For this review, take the finished solid that the model builds, in its own axes (mm). A direction names the side the tool comes from. Round coordinates to 2 decimals unless told otherwise and drop trailing zeros. Write each loop counter-clockwise with the first axis right and the second up, starting at its lowest first coordinate (ties: lowest second). Pieces come first, ordered by that corner, then holes. Notation, with made-up numbers: M -17.75,27.25 L 0.25,27.25 A18 ccw 0.25,32.25 Z; hole C 56,70.25 d3. An arc over 180 degrees is marked long. Use one line per item in the form item = value. Start each with the question number.
Item 1: Add section B-B (z = -22). State the section outline as (x, y) points.
Item 2: Add section D-D (x = -6.5). State the section outline as (y, z) points, and give its area (3 significant figures).
Item 3: For faces 4 (the flat face through (-17, -4, -15)), 5 (the cylindrical face through (0.224, 18.859, 1.203)), 6 (the cylindrical face through (0.2, 20.9, -1)), list the 3-axis set-ups (+Z, -Z, +X, -X, +Y, -Y) from which the entire face can be reached by the end or side of a thin tool; tool diameter is ignored.
Item 4: Draft analysis for pull direction Y (two halves, no side actions). For faces 1 (the flat face through (0, -16, -2)), 2 (the cylindrical face through (-1.08, -4.88, 41.52)), 3 (the flat face through (-18, 16, -17)), state which applies: released by +Y, released by -Y, zero draft, split by the parting line, or undercut.
Item 5: Add section A-A (y = 0). Count the separate pieces of the cut face and the enclosed holes in it, and give its area (3 significant figures).
Item 6: Add section C-C (y = 15). State the section outline as (x, z) points, and give its area (3 significant figures).
Item 7: For line 1 (Z direction, x = -11, y = -2); line 2 (Y direction, x = -18, z = -22); line 3 (X direction, y = 5, z = -6.5), list the stretches that pass through material, from the lowest coordinate up. Write a range as [from, to].
Item 8: For P1, Ø2, axis at x = -14, z = 13.5, coming from the -Y side; P2, Ø1, axis at x = -8, z = -1, coming from the +Y side; P3, Ø1.5, axis at x = 7.5, y = 3.5, coming from the -Z side, all flat-tipped, find the tip position at first contact; note any pin that passes through.
from build123d import *

# Parameters (mm, degrees)
SKETCH1_W                      = 32
SKETCH1_H                      = 32
BASE_FLANGE1_DEPTH             = 3
KENAR_FLAN_1_DEPTH             = 32
KENAR_FLAN_2_DEPTH             = 32
KENAR_FLAN_3_DEPTH             = 32
KENAR_FLAN_4_DEPTH             = 32
SKETCH20_R                     = 5
CUT_EXTRUDE1_DEPTH             = 82.884064384
CUT_EXTRUDE2_REACH             = 65.071
SKETCH21_R                     = 7.5
CUT_EXTRUDE2_DIRECTION_2_DEPTH = 64.071388125


# Sheet-metal steps are written as plain solids
with BuildPart() as part:
    # Sketch1 → Base-Flange1 (new body)
    with BuildSketch(Plane.XY):
        Rectangle(SKETCH1_W, SKETCH1_H)
    extrude(amount=-BASE_FLANGE1_DEPTH)

    # Kenar-Flanş1 section (across the edge) → Kenar-Flanş1 (add)
    with BuildSketch(Plane(origin=(16, 20, 0), x_dir=(0, -1, 0), z_dir=(-1, 0, 0))):
        with BuildLine():
            Line((-3, 4), (-3, 36))
            Line((-3, 36), (0, 36))
            Line((0, 36), (0, 4))
            ThreePointArc((0, 4), (1.171572875, 1.171572875), (4, 0))
            Line((4, 0), (4, -3))
            ThreePointArc((4, -3), (-0.949747468, -0.949747468), (-3, 4))
        make_face()
    extrude(amount=KENAR_FLAN_1_DEPTH)

    # Kenar-Flanş2 section (across the edge) → Kenar-Flanş2 (add)
    with BuildSketch(Plane(origin=(16, 20, 40), x_dir=(0, 0, -1), z_dir=(-1, 0, 0))):
        with BuildLine():
            Line((-3, 4), (-3, 36))
            Line((-3, 36), (0, 36))
            Line((0, 36), (0, 4))
            ThreePointArc((0, 4), (1.171572875, 1.171572875), (4, 0))
            Line((4, 0), (4, -3))
            ThreePointArc((4, -3), (-0.949747468, -0.949747468), (-3, 4))
        make_face()
    extrude(amount=KENAR_FLAN_2_DEPTH)

    # Kenar-Flanş3 section (across the edge) → Kenar-Flanş3 (add)
    with BuildSketch(Plane(origin=(-17, -16, -3), x_dir=(1, 0, 0), z_dir=(0, 1, 0))):
        with BuildLine():
            Line((-3, 1), (-3, 30))
            Line((-3, 30), (0, 30))
            Line((0, 30), (0, 1))
            ThreePointArc((0, 1), (0.292893219, 0.292893219), (1, 0))
            Line((1, 0), (1, -3))
            ThreePointArc((1, -3), (-1.828427125, -1.828427125), (-3, 1))
        make_face()
    extrude(amount=KENAR_FLAN_3_DEPTH)

    # Kenar-Flanş4 section (across the edge) → Kenar-Flanş4 (add)
    with BuildSketch(Plane(origin=(17, 16, -3), x_dir=(-1, 0, 0), z_dir=(0, -1, 0))):
        with BuildLine():
            Line((-3, 1), (-3, 30))
            Line((-3, 30), (0, 30))
            Line((0, 30), (0, 1))
            ThreePointArc((0, 1), (0.292893219, 0.292893219), (1, 0))
            Line((1, 0), (1, -3))
            ThreePointArc((1, -3), (-1.828427125, -1.828427125), (-3, 1))
        make_face()
    extrude(amount=KENAR_FLAN_4_DEPTH)

    # Sketch20 → Cut-Extrude1 (cut, through all)
    with BuildSketch(Plane.XY.offset(43)):
        Circle(SKETCH20_R)
    extrude(amount=-CUT_EXTRUDE1_DEPTH, mode=Mode.SUBTRACT)

    # Cut-Extrude2: up to this face of the body (flat: up to its plane)
    cut_extrude2_end = Plane(part.part.faces().sort_by_distance((20, 0, -18.5))[0])
    # Sketch21 → Cut-Extrude2 (cut, up to the picked face)
    with BuildSketch(Plane.ZY.offset(20), mode=Mode.PRIVATE) as cut_extrude2_sk1:
        with Locations((-22, 0)):
            Circle(SKETCH21_R)
    cut_extrude2_tool1 = split(extrude(cut_extrude2_sk1.sketch, amount=-CUT_EXTRUDE2_REACH, mode=Mode.PRIVATE), bisect_by=cut_extrude2_end, keep=Keep.BOTH, mode=Mode.PRIVATE)
    add(cut_extrude2_tool1.solids().sort_by(Axis((-20, 0, -22), (1, 0, 0)))[0], mode=Mode.SUBTRACT)

    # Sketch21 → Cut-Extrude2 direction 2 (cut)
    with BuildSketch(Plane.ZY.offset(20)):
        with Locations((-22, 0)):
            Circle(SKETCH21_R)
    extrude(amount=CUT_EXTRUDE2_DIRECTION_2_DEPTH, mode=Mode.SUBTRACT)


solid = part.part
Calculated:
q1.outline = M -20,-16 L -17,-16 L -17,-7.5 L -20,-7.5 Z; M -20,7.5 L -17,7.5 L -17,16 L -20,16 Z; M 17,-16 L 20,-16 L 20,-7.5 L 17,-7.5 Z; M 17,7.5 L 20,7.5 L 20,16 L 17,16 Z
q2.outline = M -16,-3 L 16,-3 A7 ccw 23,4 L 23,36 A7 ccw 16,43 L -16,43 L -16,40 L 16,40 A4 cw 20,36 L 20,4 A4 cw 16,0 L -16,0 Z
q2.area = 340 mm^2
q3.face_4 = -Z, +Y, -Y
q3.face_5 = +X, -X, -Y
q3.face_6 = -Z, +X, -X, +Y
q4.face_1 = released by -Y
q4.face_2 = undercut
q4.face_3 = released by +Y
q5.separate_pieces = 6
q5.enclosed_holes = 0
q5.area = 240 mm^2
q6.outline = M -20,-33 L -17,-33 L -17,-4 A1 cw -16,-3 L 16,-3 A1 cw 17,-4 L 17,-33 L 20,-33 L 20,-4 A4 ccw 16,0 L -16,0 A4 ccw -20,-4 Z; M -16,40 L 16,40 L 16,43 L -16,43 Z
q6.area = 390 mm^2
q7.line_1 = [-3, 0], [40, 43]
q7.line_2 = [-16, -7.5], [7.5, 16]
q7.line_3 = [-20, -17], [17, 20]
q8.P1 = 20
q8.P2 = 21.36
q8.P3 = -3
